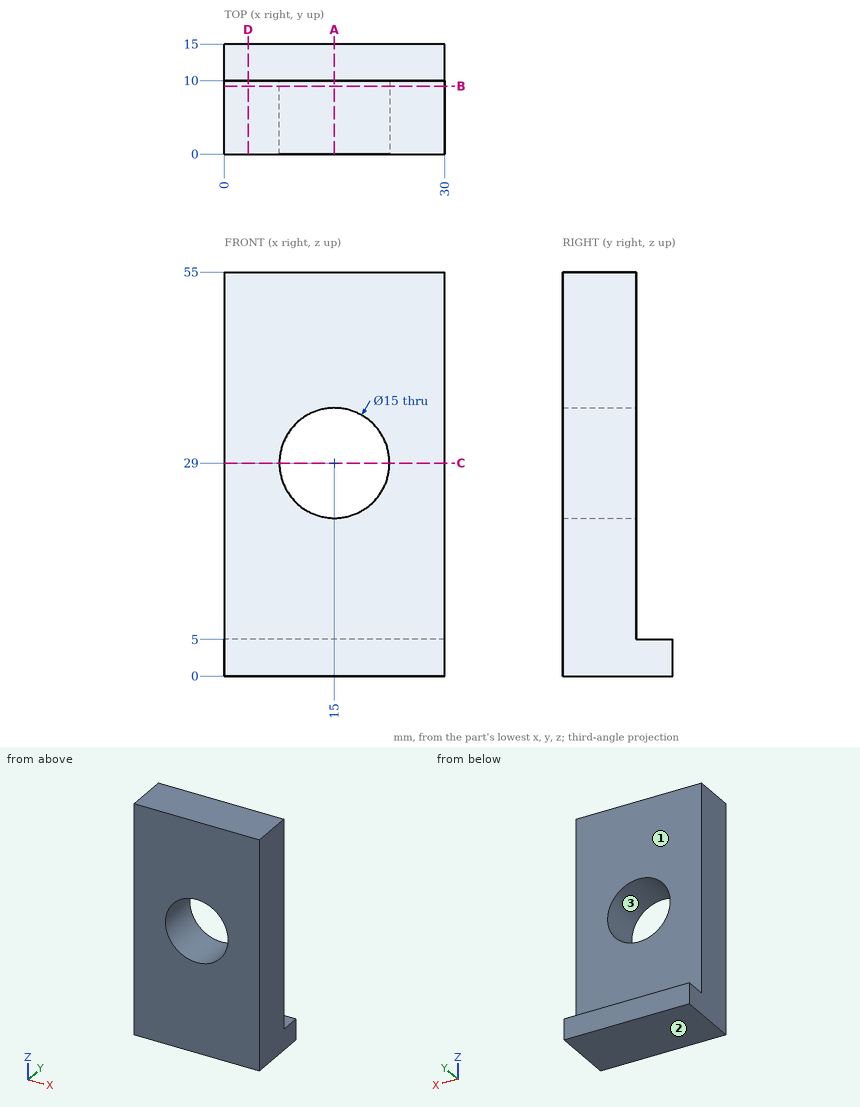
Verification items for this drawing (mm, ordinates from the low corner). Give positions to 0.01 mm unless a question says otherwise; leave off trailing zeros. Write each loop counter-clockwise with the first axis right and the second up, starting at its lowest first coordinate (ties: lowest second). Pieces come first, ordered by that corner, then holes.
1) Release check for a two-part mould opening along Z. For the marked faces 1, 2 and 3 record: released by +Z, released by -Z, zero draft, split by the parting line, or undercut.
Values follow:
face 1: zero draft
face 2: released by -Z
face 3: undercut
2) Cross-section at D-D (x = 3.25). Record the boundary of the cut face in (y, z), plus the area to 3 significant figures.
Values follow:
outline: (0, 0) - (15, 0) - (15, 5) - (10, 5) - (10, 55) - (0, 55) - close
area: 575 mm2
3) Go/stop test with flat-tipped pins: pin 1 Ø1.5 at (x, y) = (13.5, 13.5) entering from +Z; pin 2 Ø9 at (x, z) = (21, 28.5) entering from +Y. Record where each tip stops, or that it passes through.
Values follow:
pin 1: stops at z = 5
pin 2: stops at y = 10
4) Cross-section at C-C (z = 29). Record the boundary of the cut face in (x, y).
Values follow:
outline: (0, 0) - (7.5, 0) - (7.5, 10) - (0, 10) - close; (22.5, 0) - (30, 0) - (30, 10) - (22.5, 10) - close
5) Cross-section at B-B (y = 9.25). Record the boundary of the cut face in (x, z).
Values follow:
outline: (0, 0) - (30, 0) - (30, 55) - (0, 55) - close; hole circle Ø15 at (15, 29)
6) Cross-section at A-A (x = 15). Record the boundary of the cut face in (y, z), plus the area to 3 significant figures.
Values follow:
outline: (0, 0) - (15, 0) - (15, 5) - (10, 5) - (10, 21.5) - (0, 21.5) - close; (0, 36.5) - (10, 36.5) - (10, 55) - (0, 55) - close
area: 425 mm2
7) Thickness scan on line 1 (Z direction, x = 15, y = 8); line 2 (Y direction, x = 24.5, z = 44); line 3 (Z direction, x = 14.75, y = 10.25). Record the ranges inside material, lowest first.
Values follow:
line 1: z = 0 to 21.5, 36.5 to 55
line 2: y = 0 to 10
line 3: z = 0 to 5
